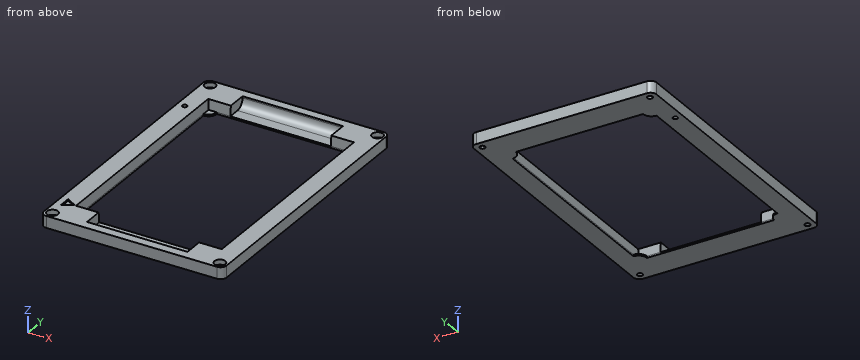
Autodesk Inventor part; units mm, degrees
ref_plane "YZ Plane" through (0, 0, 0) normal (1, 0, 0) x (0, 1, 0)
ref_plane "XZ Plane" through (0, 0, 0) normal (0, 1, 0) x (-1, 0, 0)
ref_plane "XY Plane" through (0, 0, 0) normal (0, 0, 1) x (1, 0, 0)
ref_plane "Arbeitsebene1" through (0, 0, 0) normal (0, 0, 1) x (1, 0, 0)
sketch "Skizze1" plane through (0, 0, 0) normal (0, 0, 1) x (1, 0, 0)
  line L0 (50, 77.5) -> (-50, 77.5) construction
  line L1 (-50, 77.5) -> (-50, -77.5) construction
  line L2 (-50, -77.5) -> (50, -77.5) construction
  line L3 (50, -77.5) -> (50, 77.5) construction
  line L4 (51, 82.5) -> (-51, 82.5)
  line L5 (-55, 78.5) -> (-55, -78.5)
  line L6 (-51, -82.5) -> (51, -82.5)
  line L7 (55, -78.5) -> (55, 78.5)
  circle A0 centre (50, 77.5) radius 1.6
  circle A1 centre (50, -77.5) radius 1.6
  circle A2 centre (-50, -77.5) radius 1.6
  circle A3 centre (-50, 77.5) radius 1.6
  arc A4 (55, 78.5) -> (51, 82.5) centre (51, 78.5) ccw
  arc A5 (51, -82.5) -> (55, -78.5) centre (51, -78.5) ccw
  arc A6 (-55, -78.5) -> (-51, -82.5) centre (-51, -78.5) ccw
  arc A7 (-51, 82.5) -> (-55, 78.5) centre (-51, 78.5) ccw
  line L8 (43, 64.5) -> (43, -64.5)
  line L9 (-43, -64.5) -> (-43, 64.5)
  line L10 (-43, 63.5) -> (-43, 64.5)
  line L11 (-43, 64.5) -> (43, 64.5)
  line L12 (43, 64.5) -> (43, 74.0537)
  line L13 (-43, -64.5) -> (43, -64.5)
  circle A8 centre (-43, 64.5) radius 5
  circle A9 centre (43, 64.5) radius 5
  circle A10 centre (43, -64.5) radius 5
  circle A11 centre (-43, -64.5) radius 5
  point P0 (0, 0)
  point P1 (-43, -59.5)
  point P2 (-43, 59.5)
  point P3 (-38, 64.5)
  point P4 (38, 64.5)
  point P5 (43, 59.5)
  point P6 (43, -59.5)
  point P7 (38, -64.5)
  point P8 (-38, -64.5)
  dimension "d1" = 3.2
  dimension "d2" = 3.2
  dimension "d3" = 3.2
  dimension "d4" = 3.2
  dimension "d5" = 4
  dimension "d6" = 86
  dimension "d10" = 10
  dimension "d11" = 10
  dimension "d12" = 10
  dimension "d13" = 10
  dimension "d31" = 43
  dimension "d32" = 129
  dimension "d33" = 100
  dimension "d34" = 155
  dimension "d35" = 64.5
  dimension "d36" = 55
  dimension "d37" = 110
  dimension "d38" = 165
  dimension "d39" = 82.5
extrude "Extrusion1" add sketch "Skizze1" along normal blind 1 contours A4 L7 A5 L6 A6 L5 A7 L4 | L12 A9 L8 | L8 A9 L11 | L11 A9 L12 | A10 L13 L8 | L8 L13 A10 | A8 L9 L11 | L11 L9 A8 | A11 L9 L13 | L13 L9 A11
sketch "Skizze2" plane through (0, 0, 1) normal (0, 0, 1) x (1, 0, 0)
  arc A0 (-51, 82.5) -> (-55, 78.5) centre (-51, 78.5) ccw
  line L0 (-55, 78.5) -> (-55, -78.5)
  arc A1 (-55, -78.5) -> (-51, -82.5) centre (-51, -78.5) ccw
  line L1 (-51, -82.5) -> (51, -82.5)
  arc A2 (51, -82.5) -> (55, -78.5) centre (51, -78.5) ccw
  line L2 (55, -78.5) -> (55, 78.5)
  arc A3 (55, 78.5) -> (51, 82.5) centre (51, 78.5) ccw
  line L3 (51, 82.5) -> (-51, 82.5)
  arc A4 (-38, -64.5) -> (-43, -59.5) centre (-43, -64.5) ccw
  line L4 (-43, -59.5) -> (-43, 59.5)
  arc A5 (-43, 59.5) -> (-38, 64.5) centre (-43, 64.5) ccw
  line L5 (-38, 64.5) -> (38, 64.5)
  arc A6 (38, 64.5) -> (43, 59.5) centre (43, 64.5) ccw
  line L6 (43, 59.5) -> (43, -59.5)
  arc A7 (43, -59.5) -> (38, -64.5) centre (43, -64.5) ccw
  line L7 (38, -64.5) -> (-38, -64.5)
  circle A8 centre (-50, 77.5) radius 1.6
  circle A9 centre (-50, -77.5) radius 1.6
  circle A10 centre (50, -77.5) radius 1.6
  circle A11 centre (50, 77.5) radius 1.6
  line L8 (-43, 64.5) -> (43, 64.5)
  line L9 (43, 64.5) -> (43, -64.5)
  line L10 (43, -64.5) -> (-43, -64.5)
  line L11 (-43, -64.5) -> (-43, 64.5)
  point P0 (-43, 59.5)
  point P1 (43, -59.5)
  point P2 (38, -64.5)
  point P3 (-43, -59.5)
extrude "Extrusion2" add sketch "Skizze2" along normal blind 6 draft -5
sketch "Skizze3" plane through (0, 0, 7) normal (0, 0, 1) x (1, 0, 0)
  line L0 (-44.539, -64.7031) -> (-50.539, -68.1672)
  line L1 (-50.539, -68.1672) -> (-50.539, -61.239)
  line L2 (-50.539, -61.239) -> (-44.539, -64.7031)
  line L3 (39.5249, 74.6999) -> (39.5249, -55.3499)
  point P0 (0, 0)
  point P1 (-48.539, -64.7031)
  dimension "d23" = 6
extrude "Extrusion3" cut sketch "Skizze3" against normal blind 1
sketch "Skizze4" plane through (0, 0, 7) normal (0, 0, 1) x (1, 0, 0)
  line L0 (-44.539, -64.7031) -> (-50.539, -68.1672)
  line L1 (-50.539, -61.239) -> (-44.539, -64.7031)
  circle A0 centre (-50, 77.5) radius 2.1249
  circle A1 centre (-50, -77.5) radius 2.1249
  circle A2 centre (50, -77.5) radius 2.1249
  circle A3 centre (50, 77.5) radius 2.1249
  line L2 (-54.4751, -78.5) -> (-54.4751, 78.5)
  arc A4 (-54.4751, -78.5) -> (-51, -81.9751) centre (-51, -78.5) ccw
  line L3 (51, -81.9751) -> (-51, -81.9751)
  arc A5 (51, -81.9751) -> (54.4751, -78.5) centre (51, -78.5) ccw
  line L4 (54.4751, 78.5) -> (54.4751, -78.5)
  arc A6 (54.4751, 78.5) -> (51, 81.9751) centre (51, 78.5) ccw
  line L5 (-51, 81.9751) -> (51, 81.9751)
  arc A7 (-51, 81.9751) -> (-54.4751, 78.5) centre (-51, 78.5) ccw
  circle A8 centre (-50, -77.5) radius 1.6
  circle A9 centre (50, -77.5) radius 1.6
  circle A10 centre (50, 77.5) radius 1.6
  circle A11 centre (-50, 77.5) radius 1.6
  line L6 (-50.539, -68.1672) -> (-50.539, -61.239)
  point P0 (0, 0)
hole "Bohrung1" at (-50, -77.5, 7) at (50, -77.5, 7) at (50, 77.5, 7) at (-50, 77.5, 7) direction (0, 0, -1) diameter 3.2 end through all counterbore diameter 6.5 counterbore depth 3
sketch "Skizze5" plane through (0, 0, 0) normal (1, 0, 0) x (0, 1, 0)
  line L0 (64.5, 1) -> (65.0249, 7)
  line L1 (64.5, 1) -> (71.5, 1)
  line L2 (76.5, 6) -> (76.5, 16)
  line L3 (76.5, 16) -> (64.5, 16)
  line L4 (64.5, 16) -> (64.5, 1)
  line L5 (-64.5, 0) -> (-64.5, 1)
  line L6 (-64.5, 1) -> (-71.5, 1)
  line L7 (-76.5, 6) -> (-76.5, 12.183)
  line L8 (-76.5, 12.183) -> (-64.5, 12.183)
  line L9 (-64.5, 12.183) -> (-64.5, 1)
  arc A0 (-76.5, 6) -> (-71.5, 1) centre (-71.5, 6) ccw
  arc A1 (71.5, 1) -> (76.5, 6) centre (71.5, 6) ccw
  point P0 (0, 0)
  point P1 (76.5, 1)
  dimension "d40" = 12
  dimension "d41" = 15
  dimension "d42" = 12
  dimension "d43" = 5
extrude "Extrusion4" cut sketch "Skizze5" along normal mid plane 60
sketch "Skizze6" plane through (0, 0, 7) normal (0, 0, 1) x (1, 0, 0)
  circle A0 centre (-50, 77.5) radius 1.8625
  line L0 (-43.5249, -65.0249) -> (-43.5249, 65.0249)
  line L1 (-43.5249, 65.0249) -> (-37.8681, 65.0249) construction
  circle A1 centre (-50, 52.5) radius 1.4
  point P0 (0, 0)
  dimension "d48" = 2.8
  dimension "d51" = 25
extrude "Extrusion5" cut sketch "Skizze6" against normal blind 60 contours A1
sketch "Skizze7" plane through (0, 0, 7) normal (0, 0, 1) x (1, 0, 0)
  circle A0 centre (-50, 52.5) radius 1.4
  line L0 (-54.4751, -78.5) -> (-54.4751, 78.5)
  arc A1 (-54.4751, -78.5) -> (-51, -81.9751) centre (-51, -78.5) ccw
  line L1 (51, -81.9751) -> (-51, -81.9751)
  arc A2 (51, -81.9751) -> (54.4751, -78.5) centre (51, -78.5) ccw
  line L2 (54.4751, 78.5) -> (54.4751, -78.5)
  arc A3 (54.4751, 78.5) -> (51, 81.9751) centre (51, 78.5) ccw
  line L3 (-51, 81.9751) -> (51, 81.9751)
  arc A4 (-51, 81.9751) -> (-54.4751, 78.5) centre (-51, 78.5) ccw
  line L4 (-44.539, -64.7031) -> (-50.539, -68.1672)
  line L5 (-50.539, -68.1672) -> (-50.539, -61.239)
  line L6 (-50.539, -61.239) -> (-44.539, -64.7031)
  circle A5 centre (-50, 77.5) radius 3.25
  circle A6 centre (50, -77.5) radius 3.25
  circle A7 centre (-50, -77.5) radius 3.25
  circle A8 centre (50, 77.5) radius 3.25
  line L7 (30, -65.0249) -> (30, -76.5)
  line L8 (30, -76.5) -> (-30, -76.5)
  line L9 (-30, -76.5) -> (-30, -65.0249)
  line L10 (-30, -65.0249) -> (-43.5249, -65.0249)
  line L11 (-43.5249, -65.0249) -> (-43.5249, 65.0249)
  line L12 (-43.5249, 65.0249) -> (-30, 65.0249)
  line L13 (-30, 65.0249) -> (-30, 76.5)
  line L14 (-30, 76.5) -> (30, 76.5)
  line L15 (30, 76.5) -> (30, 65.0249)
  line L16 (30, 65.0249) -> (43.5249, 65.0249)
  line L17 (43.5249, 65.0249) -> (43.5249, -65.0249)
  line L18 (43.5249, -65.0249) -> (30, -65.0249)
  line L19 (-50, -81.5) -> (50, -81.5)
  line L20 (54, -77.5) -> (54, 77.5)
  line L21 (50, 81.5) -> (-50, 81.5)
  line L22 (-54, 77.5) -> (-54, -77.5)
  line L23 (-54, -81.5) -> (54, 81.5) construction
  line L24 (54, -81.5) -> (-54, 81.5) construction
  arc A9 (54, 77.5) -> (50, 81.5) centre (50, 77.5) ccw
  arc A10 (-50, 81.5) -> (-54, 77.5) centre (-50, 77.5) ccw
  arc A11 (-54, -77.5) -> (-50, -81.5) centre (-50, -77.5) ccw
  arc A12 (50, -81.5) -> (54, -77.5) centre (50, -77.5) ccw
  point P0 (0, 0)
  dimension "d52" = 108
  dimension "d53" = 163
  dimension "d54" = 4
extrude "Extrusion6" cut sketch "Skizze7" against normal blind 10 contours A0 | L0 A4 L3 A3 L2 A2 L1 A1 | L4 L5 L6 | A5 | A6 | A7 | A8 | L7 L8 L9 L10 L11 L12 L13 L14 L15 L16 L17 L18 | A11 L22 A10 L21 A9 L20 A12 L19 keep common part
equation "\"d11\" = d10"
equation "\"d12\" = d10"
equation "\"d13\" = d10"
properties part number "30_xystage_gp-010b_adapter_multiwellplate"
Read the model definition and answer for the solid it produces. Units are mm, in the model's axes. Coordinates: 2 decimals unless noted, no trailing zeros. Write each loop counter-clockwise with the first axis right and the second up, starting at its lowest first coordinate (ties: lowest second). Pieces come first, ordered by that corner, then holes. Notation, with made-up numbers: (48, 31.25) -> (89, 31.25) arc R35 ccw to (89, 66.25) -> close; hole circle Ø6 at (40, -27.75). An arc over 180 degrees is marked (long way). Return JSON: item names as keys, results as strings.
(1) The part is cut by section A-A on y = 42. Give the vertices of the cut face in (x, z), then the cut area to 3 significant figures.
Answers below:
{"outline": "(-54.48, 0) -> (-43, 0) -> (-43, 1) -> (-43.52, 7) -> (-54.48, 7) -> close; (43, 0) -> (54.48, 0) -> (54.48, 7) -> (43.52, 7) -> (43, 1) -> close", "area": "158 mm^2"}
(2) The part is cut by section D-D on x = 24. Give the vertices of the cut face in (y, z), then the cut area to 3 significant figures.
Answers below:
{"outline": "(-81.98, 0) -> (-64.5, 0) -> (-64.5, 1) -> (-71.5, 1) arc R5 cw to (-76.5, 6) -> (-76.5, 7) -> (-81.98, 7) -> close; (64.5, 0) -> (81.98, 0) -> (81.98, 7) -> (76.5, 7) -> (76.5, 6) arc R5 cw to (71.5, 1) -> (64.5, 1) -> close", "area": "111 mm^2"}
(3) Each of these flat-tipped pins is pushed along its axis until it touches: P1, Ø2.5, axis at x = -50, y = 52.5, coming from the -Z side; P2, Ø5, axis at x = 51.5, y = -78, coming from the +Z side; P3, Ø2, axis at x = -11.5, y = -68, coming from the +Z side; P4, Ø5, axis at x = 50, y = 77.5, coming from the +Z side. Where does it stop, or does it pass through?
Answers below:
{"P1": "through", "P2": "z = 7", "P3": "z = 1", "P4": "z = 4"}
(4) The part is cut by section C-C on y = 67.5. Give the vertices of the cut face in (x, z), then the cut area to 3 significant figures.
Answers below:
{"outline": "(-54.48, 0) -> (54.48, 0) -> (54.48, 7) -> (30, 7) -> (30, 1) -> (-30, 1) -> (-30, 7) -> (-54.48, 7) -> close", "area": "403 mm^2"}
(5) Consider line 1 along X through (y, z) = (-77.5, 4.75); line 2 along X through (y, z) = (-77.5, 0.4); line 3 along Y through (x, z) = (-50, 4.25). Determine where each line is inside the solid, lowest interval first. Write a range as from..to.
Answers below:
{"line 1": "-54.48..-53.25, -46.75..46.75, 53.25..54.48", "line 2": "-54.48..-51.6, -48.4..48.4, 51.6..54.48", "line 3": "-81.98..-80.75, -74.25..51.1, 53.9..74.25, 80.75..81.98"}
(6) The part is cut by section B-B on x = -36. Give the vertices of the cut face in (y, z), then the cut area to 3 significant figures.
Answers below:
{"outline": "(-81.98, 0) -> (-64.5, 0) -> (-64.5, 1) -> (-65.02, 7) -> (-81.98, 7) -> close; (64.5, 0) -> (81.98, 0) -> (81.98, 7) -> (65.02, 7) -> (64.5, 1) -> close", "area": "242 mm^2"}
